```python
from build123d import *

# Parameters (mm, degrees)
F0_W           = 127
F0_H           = 127
F1_DEPTH       = 9.144
F3_D           = 15.24
F3_CBORE_D     = 15.24
F3_CBORE_DEPTH = 50.8
F4_D           = 15.24
F4_CBORE_D     = 15.24
F4_CBORE_DEPTH = 50.8
F5_D           = 15.24
F5_CBORE_D     = 15.24
F5_CBORE_DEPTH = 50.8
F6_D           = 15.24
F6_CBORE_D     = 15.24
F6_CBORE_DEPTH = 50.8


with BuildPart() as f1:
    # F0 (on Top) → F1 (new body)
    with BuildSketch(Plane.XY):
        with Locations((63.5, -63.5)):
            Rectangle(F0_W, F0_H)
    extrude(amount=F1_DEPTH)

    # F3 (through all)
    with Locations(Plane.XY.offset(9.144)):
        with Locations((63.5, -12.7)):
            CounterBoreHole(F3_D / 2, F3_CBORE_D / 2, F3_CBORE_DEPTH)

    # F4 (through all)
    with Locations(Plane.XY.offset(9.144)):
        with Locations((12.7, -63.5)):
            CounterBoreHole(F4_D / 2, F4_CBORE_D / 2, F4_CBORE_DEPTH)

    # F5 (through all)
    with Locations(Plane.XY.offset(9.144)):
        with Locations((63.5, -114.3)):
            CounterBoreHole(F5_D / 2, F5_CBORE_D / 2, F5_CBORE_DEPTH)

    # F6 (through all)
    with Locations(Plane.XY.offset(9.144)):
        with Locations((114.3, -63.5)):
            CounterBoreHole(F6_D / 2, F6_CBORE_D / 2, F6_CBORE_DEPTH)


solid = f1.part
```
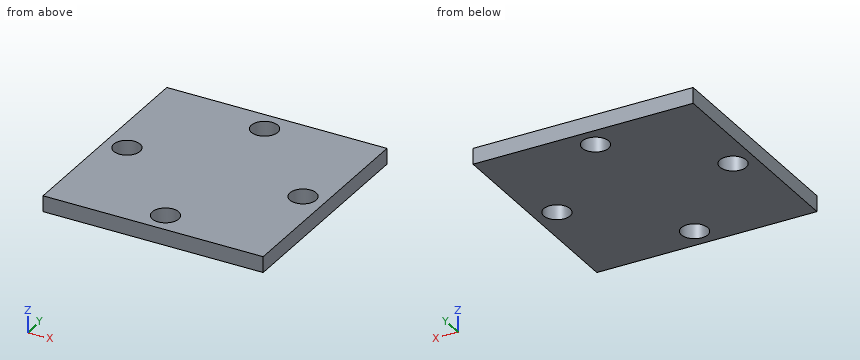
Can you work these out from the model? Positions are in its coordinate system, mm. Round coordinates to 2 decimals unless told otherwise and drop trailing zeros. Order: outer loops, then holes, each group sorted by start corner. A loop starts at its lowest first (then second) coordinate and runs counter-clockwise, first axis right, second up. Notation, with made-up numbers: (67.5, 31.25) -> (85.5, 31.25) arc R33 cw to (85.5, 61.25) -> close; hole circle Ø6 at (2, -32.75). An arc over 180 degrees is marked (long way). Return JSON: item names as keys, results as strings. Group by question number.
1. If we section it at D-D, the plane x = 12.7: Write out the boundary of the cut face in (y, z).
2. If we section it at C-C, the plane y = -63.5: Write out the boundary of the cut face in (x, z), then the cut area to 3 significant figures.
3. I need wall thicknesses on line 1 (X direction, y = -63.5, z = 4.25); line 2 (Y direction, x = 63.5, z = 3.75); line 3 (Y direction, x = 114.3, z = 3.5). Which ranges of each line are inside material? Lowest first, please. Write a range as [from, to].
4. If we section it at A-A, the plane y = -12.7: Write out the boundary of the cut face in (x, z).
5. If we section it at B-B, the plane x = 63.5: Write out the boundary of the cut face in (y, z).
6. Will this pin go through, and if not, where does the flat tip stop? pin 1 (13.5 mm diameter, centred on x = 114.3, y = -63.5, fed in from +Z).
Output values:
{
 "1": {"outline": "(-127, 0) -> (-71.12, 0) -> (-71.12, 9.14) -> (-127, 9.14) -> close; (-55.88, 0) -> (0, 0) -> (0, 9.14) -> (-55.88, 9.14) -> close"},
 "2": {"outline": "(0, 0) -> (5.08, 0) -> (5.08, 9.14) -> (0, 9.14) -> close; (20.32, 0) -> (106.68, 0) -> (106.68, 9.14) -> (20.32, 9.14) -> close; (121.92, 0) -> (127, 0) -> (127, 9.14) -> (121.92, 9.14) -> close", "area": "883 mm²"},
 "3": {"line 1": "[0, 5.08], [20.32, 106.68], [121.92, 127]", "line 2": "[-127, -121.92], [-106.68, -20.32], [-5.08, 0]", "line 3": "[-127, -71.12], [-55.88, 0]"},
 "4": {"outline": "(0, 0) -> (55.88, 0) -> (55.88, 9.14) -> (0, 9.14) -> close; (71.12, 0) -> (127, 0) -> (127, 9.14) -> (71.12, 9.14) -> close"},
 "5": {"outline": "(-127, 0) -> (-121.92, 0) -> (-121.92, 9.14) -> (-127, 9.14) -> close; (-106.68, 0) -> (-20.32, 0) -> (-20.32, 9.14) -> (-106.68, 9.14) -> close; (-5.08, 0) -> (0, 0) -> (0, 9.14) -> (-5.08, 9.14) -> close"},
 "6": {"pin 1": "through"}
}
